Source: three-view drawing plus pictorial views. Frame: mm from the lowest corner of the part. Give positions to 0.01 mm unless a question says otherwise; leave off trailing zeros. Loops run counter-clockwise (first coordinate to the right, second up) from the corner with the lowest first, then second, coordinate; pieces in that order, holes last. Notation, with made-up numbers: (20.25, 49.5) - (36.25, 49.5) arc R19 cw to (36.25, 85.5) - close; hole circle Ø4 at (17, -30.5). An arc over 180 degrees is marked (long way). Answer as a JSON object with one key per item and string values.
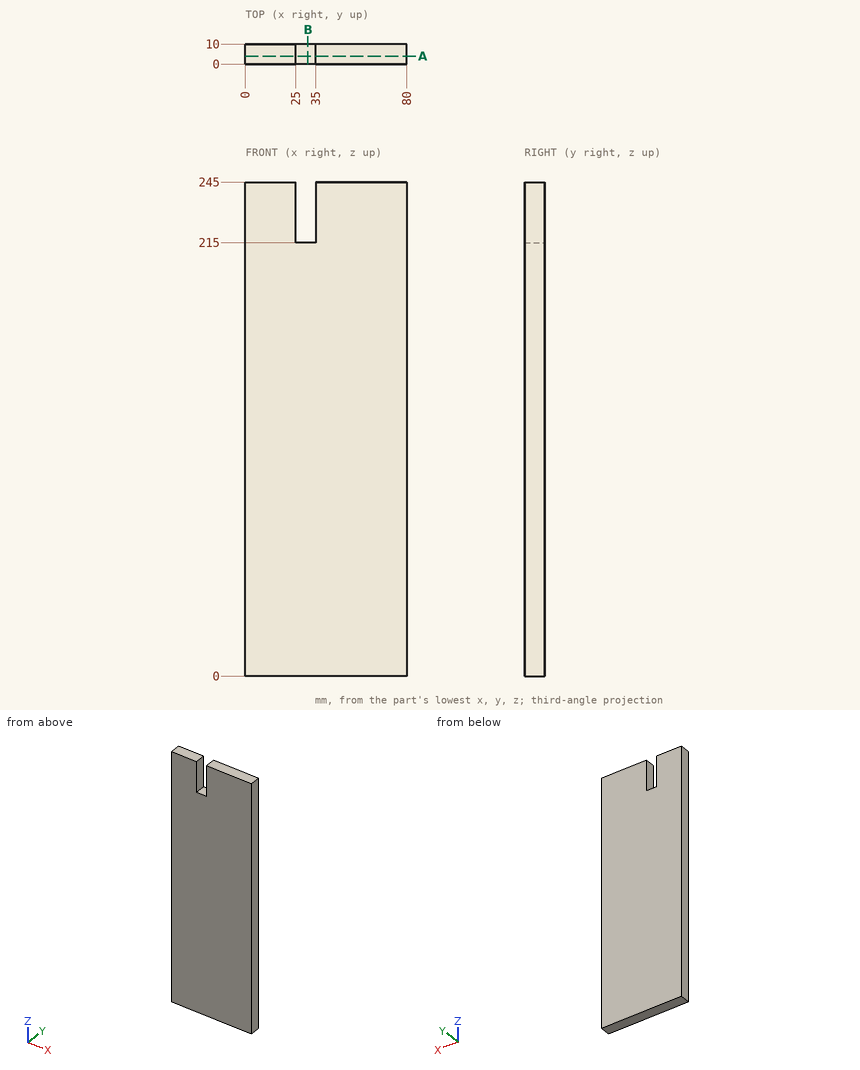
Item 1: Cut plane B-B (x = 31). Return loops of the section in (y, z), then the cut area to 3 significant figures.
Geometry check:
{"outline": "(0, 0) - (10, 0) - (10, 215) - (0, 215) - close", "area": "2,150 mm2"}
Item 2: Material intervals for line 1 (X direction, y = 1, z = 220.5); line 2 (Z direction, x = 32, y = 8.5), sorted ascending. Write a range as [from, to].
Geometry check:
{"line 1": "x = [0, 25], [35, 80]", "line 2": "z = [0, 215]"}
Item 3: Contact query for a flat-ended pin moving along its axis: P1, Ø5, axis at x = 30, y = 6, coming from the +Z side. Output: stop coordinate, or through.
Geometry check:
{"P1": "stops at z = 215"}
Item 4: Cut plane A-A (y = 4). Return loops of the section in (x, z).
Geometry check:
{"outline": "(0, 0) - (80, 0) - (80, 245) - (35, 245) - (35, 215) - (25, 215) - (25, 245) - (0, 245) - close"}
